For this review, take the finished solid that the model builds, in its own axes (mm). Coordinates: 2 decimals unless noted, no trailing zeros. Order: outer loops, then holes, each group sorted by start corner. A loop starts at its lowest first (then second) coordinate and runs counter-clockwise, first axis right, second up.
from build123d import *

# Parameters (mm, degrees)
BOSS_EXTRUDE1_DEPTH = 3
SKETCH2_W           = 15
SKETCH2_H           = 3
CUT_EXTRUDE1_DEPTH  = 3


with BuildPart() as part:
    # Sketch1 → Boss-Extrude1 (new body)
    with BuildSketch(Plane(origin=(0, 0, 0), x_dir=(1, 0, 0), z_dir=(0, 1, 0))):
        Polygon((-35, -35), (-17.5, -35), (-17.5, -38), (17.5, -38), (17.5, -35), (35, -35), (35, -17.5), (38, -17.5), (38, 17.5), (35, 17.5), (35, 35), (17.5, 35), (17.5, 38), (-17.5, 38), (-17.5, 35), (-35, 35), (-35, 17.5), (-38, 17.5), (-38, -17.5), (-35, -17.5), align=None)
    extrude(amount=BOSS_EXTRUDE1_DEPTH)

    # Sketch2 → Cut-Extrude1 (cut)
    with BuildSketch(Plane(origin=(0, 3, 0), x_dir=(1, 0, 0), z_dir=(0, 1, 0))):
        Rectangle(SKETCH2_W, SKETCH2_H)
    extrude(amount=-CUT_EXTRUDE1_DEPTH, mode=Mode.SUBTRACT)


solid = part.part
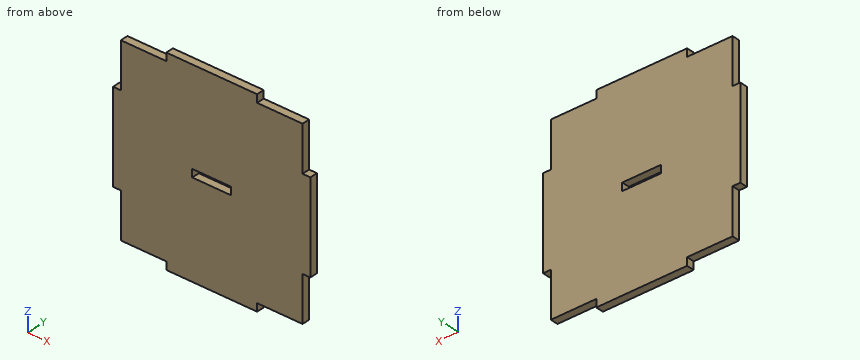
1. Take a section at B-B, the plane y = 1.25. Give the boundary of the cut face in (x, z), plus the area to 4 significant figures.
Answer below:
outline: (-38, -17.5) - (-35, -17.5) - (-35, -35) - (-17.5, -35) - (-17.5, -38) - (17.5, -38) - (17.5, -35) - (35, -35) - (35, -17.5) - (38, -17.5) - (38, 17.5) - (35, 17.5) - (35, 35) - (17.5, 35) - (17.5, 38) - (-17.5, 38) - (-17.5, 35) - (-35, 35) - (-35, 17.5) - (-38, 17.5) - close; hole (-7.5, -1.5) - (7.5, -1.5) - (7.5, 1.5) - (-7.5, 1.5) - close
area: 5,275 mm2
2. Take a section at D-D, the plane x = -28. Give the boundary of the cut face in (y, z).
Answer below:
outline: (0, -35) - (3, -35) - (3, 35) - (0, 35) - close
3. Clearance check with flat-ended pins moving along their axes: pin 1 Ø1.5 at (x, y) = (-24, 1.5) entering from -Z; pin 2 Ø0.9 at (y, z) = (1, 36.5) entering from +X; pin 3 Ø0.9 at (x, y) = (-37, 2) entering from +Z. State where each tip first meets the part, or that it passes through.
Answer below:
pin 1: stops at z = -35
pin 2: stops at x = 17.5
pin 3: stops at z = 17.5
4. Take a section at C-C, the plane z = 27.5. Give the boundary of the cut face in (x, y).
Answer below:
outline: (-35, 0) - (35, 0) - (35, 3) - (-35, 3) - close
5. To check wall thickness, follow L1, parallel to Z at x = 2, y = 1.25; L2, parallel to Z at x = 23, y = 1.9. State the ranges of each line that lie inside material, in increasing order.
Answer below:
L1: z = -38 to -1.5, 1.5 to 38
L2: z = -35 to 35
6. Take a section at A-A, the plane x = -3.5. Give the boundary of the cut face in (y, z), plus the area to 3 significant figures.
Answer below:
outline: (0, -38) - (3, -38) - (3, -1.5) - (0, -1.5) - close; (0, 1.5) - (3, 1.5) - (3, 38) - (0, 38) - close
area: 219 mm2
